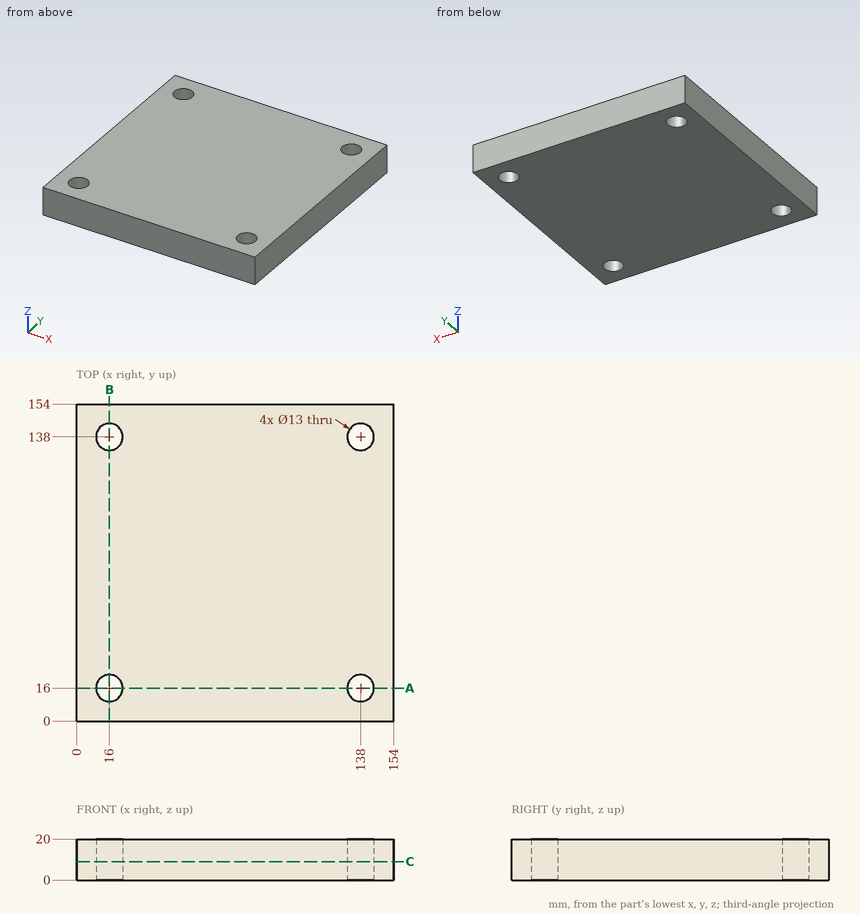
Drawing for the job (mm, zero at the part's lowest x, y, z). Give positions to 0.01 mm unless a question says otherwise; leave off trailing zeros. Write each loop counter-clockwise with the first axis right and the second up, starting at its lowest first coordinate (ties: lowest second). Pieces come first, ordered by that corner, then holes. Notation, with made-up numbers: M -5,82.5 L 15,82.5 A23 cw 15,112.5 Z; hole C 58,26 d9. An arc over 180 degrees is marked long. Return JSON: item names as keys, results as strings. Group by question number.
(1) Band-saw the part on C-C (z = 9). Give the cut face in (x, y).
(2) Band-saw the part on A-A (y = 16). Give the cut face in (x, z), and give its area (3 significant figures).
(3) Drill centre lines: L1, parallel to Y at x = 138, z = 6; L2, parallel to X at y = 18, z = 12; L3, parallel to Y at x = 17.5, z = 12.5. Where is each one in solid material? Low to high. Write a range as [from, to].
(4) Flat gauge pin, fed straight in: pin 1 Ø10.5 at (x, y) = (16, 16) entering from +Z. Where does the tip first touch, or does it go through?
Entries:
{
 "1": {"outline": "M 0,0 L 154,0 L 154,154 L 0,154 Z; hole C 16,16 d13; hole C 16,138 d13; hole C 138,16 d13; hole C 138,138 d13"},
 "2": {"outline": "M 0,0 L 9.5,0 L 9.5,20 L 0,20 Z; M 22.5,0 L 131.5,0 L 131.5,20 L 22.5,20 Z; M 144.5,0 L 154,0 L 154,20 L 144.5,20 Z", "area": "2,560 mm^2"},
 "3": {"L1": "y = [0, 9.5], [22.5, 131.5], [144.5, 154]", "L2": "x = [0, 9.82], [22.18, 131.82], [144.18, 154]", "L3": "y = [0, 9.68], [22.32, 131.68], [144.32, 154]"},
 "4": {"pin 1": "passes through"}
}
